```python
from build123d import *

# Parameters (mm, degrees)
SKETCH1_W           = 15.875
SKETCH1_H           = 83.83778
SKETCH1_W_2         = 3.175
SKETCH1_H_2         = 6.604
BOSS_EXTRUDE1_DEPTH = 2.38125
SKETCH2_W           = 5.42671
SKETCH2_H           = 83.83778
SKETCH2_W_2         = 23.424388
BOSS_EXTRUDE2_DEPTH = 2.38125
SKETCH3_W           = 3.175
SKETCH3_H           = 64.78778
SKETCH3_H_2         = 6.35
CUT_EXTRUDE2_DEPTH  = 90.543351098
BOSS_EXTRUDE4_DEPTH = 2.38125
FILLET1_R           = 10.16
CUT_EXTRUDE5_DEPTH  = 109.143259408


with BuildPart() as part:
    # Sketch1 → Boss-Extrude1 (new body)
    with BuildSketch(Plane.XY):
        with Locations((0, 41.91889)):
            Rectangle(SKETCH1_W, SKETCH1_H)
        with Locations((-1.27, 68.08976095)):
            Rectangle(SKETCH1_W_2, SKETCH1_H_2, mode=Mode.SUBTRACT)
    extrude(amount=BOSS_EXTRUDE1_DEPTH)

    # Sketch2 → Boss-Extrude2 (add)
    with BuildSketch(Plane.XY):
        with Locations((10.650855, 41.91889)):
            Rectangle(SKETCH2_W, SKETCH2_H)
        with Locations((-19.649694, 41.91889)):
            Rectangle(SKETCH2_W_2, SKETCH2_H)
    extrude(amount=BOSS_EXTRUDE2_DEPTH)

    # Sketch3 → Cut-Extrude2 (cut, through all)
    with BuildSketch(Plane.XY):
        with Locations((-29.774388, 51.44389)):
            Rectangle(SKETCH3_W, SKETCH3_H)
        with Locations((11.77671, 51.44389)):
            Rectangle(SKETCH3_W, SKETCH3_H)
        with Locations((-29.774388, 3.175)):
            Rectangle(SKETCH3_W, SKETCH3_H_2)
        with Locations((11.77671, 3.175)):
            Rectangle(SKETCH3_W, SKETCH3_H_2)
    extrude(amount=CUT_EXTRUDE2_DEPTH, mode=Mode.SUBTRACT)

    # Sketch5 → Boss-Extrude4 (add)
    with BuildSketch(Plane.XY):
        Polygon((-28.186888, 0), (-28.186888, -6.35), (-68.268007503, -19.717143922), (-68.268007503, -32.282068045), (50.270329503, -32.282068045), (50.270329503, -19.717143922), (10.18921, -6.35), (10.18921, 0), align=None)
    extrude(amount=BOSS_EXTRUDE4_DEPTH)

    # Fillet1
    fillet1_edges = [part.edges().sort_by_distance(p)[0] for p in [
        (-28.186888, -6.35, 1.190625),
        (-68.268007503, -19.717143922, 1.190625),
        (50.270329503, -19.717143922, 1.190625),
        (10.18921, -6.35, 1.190625),
    ]]
    fillet(fillet1_edges, radius=FILLET1_R)

    # Sketch6 → Cut-Extrude5 (cut, through all)
    with BuildSketch(Plane.XY):
        Polygon((-36.518007503, -32.282068045), (-36.518007503, -27.870697677), (-39.076507827, -27.870697677), (-39.076507827, -25.312197354), (-36.518007503, -25.312197354), (-36.518007503, -23.233415841), (-33.479788369, -23.233415841), (-33.479788369, -25.312197354), (-30.921288046, -25.312197354), (-30.921288046, -27.870697677), (-33.479788369, -27.870697677), (-33.479788369, -32.282068045), align=None)
        Polygon((15.482110369, -32.282068045), (15.482110369, -27.870697677), (12.923610046, -27.870697677), (12.923610046, -25.312197354), (15.482110369, -25.312197354), (15.482110369, -23.233415841), (18.520329503, -23.233415841), (18.520329503, -25.312197354), (21.078829827, -25.312197354), (21.078829827, -27.870697677), (18.520329503, -27.870697677), (18.520329503, -32.282068045), align=None)
    extrude(amount=CUT_EXTRUDE5_DEPTH, mode=Mode.SUBTRACT)


solid = part.part
```
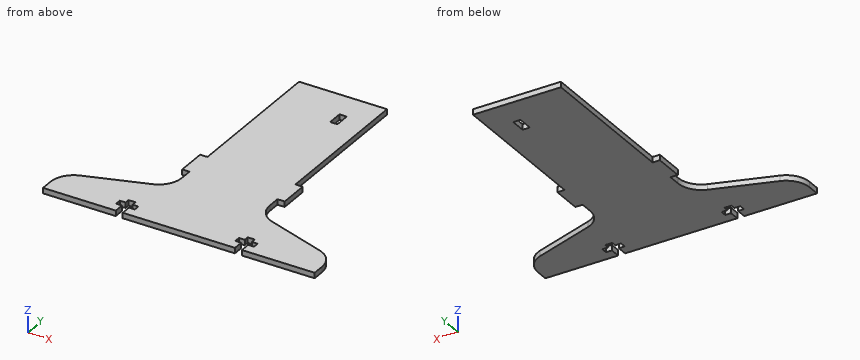
Input: part model. Units: mm. Frame: model coordinates. Give positions to 0.01 mm unless a question says otherwise; leave off trailing zeros. Write each loop counter-clockwise with the first axis right and the second up, starting at its lowest first coordinate (ties: lowest second). Pieces come first, ordered by that corner, then holes. Notation, with made-up numbers: (76.25, 73.5) - (89.25, 73.5) arc R9 cw to (89.25, 89.5) - close; hole circle Ø4 at (-34, 15). An arc over 180 degrees is marked (long way). Write item = value, one per line. Start each with the question number.
1. Ray query, L1, parallel to X at y = -27, z = 0.55; L2, parallel to X at y = 69.5, z = 1.35; L3, parallel to X at y = 15, z = 2.05. Return the intervals inside material, ascending.
2. First-contact query: pin 1 Ø1.2 at (x, z) = (-35, 1.5) entering from -Y; pin 2 Ø1.2 at (y, z) = (68, 1.5) entering from +X; pin 3 Ø0.7 at (y, z) = (-26, 1.5) entering from -X. Flat tips, straight axial feed; report the tip coordinate or a pass-through.
3. Section query A-A, the plane y = 13.5. Output: boundary loops of the cut face in (x, z), then the cut area to 3 significant figures.
4. Section query B-B, the plane x = -41.5. Output: boundary loops of the cut face in (y, z).
Check sheet entries:
q1.L1 = -68.27 to -39.08, -30.92 to 12.92, 21.08 to 50.27
q1.L2 = -28.19 to -2.86, 0.32 to 10.19
q1.L3 = -31.36 to 13.36
q2.pin_1 = -23.23
q2.pin_2 = 10.19
q2.pin_3 = -68.24
q3.outline = (-31.36, 0) - (13.36, 0) - (13.36, 2.38) - (-31.36, 2.38) - close
q3.area = 107 mm2
q4.outline = (-32.28, 0) - (-10.79, 0) - (-10.79, 2.38) - (-32.28, 2.38) - close
